For this review, take the finished solid that the model builds, in its own axes (mm). A direction names the side the tool comes from. Round coordinates to 2 decimals unless told otherwise and drop trailing zeros. Order: outer loops, then holes, each group sorted by start corner. A loop starts at its lowest first (then second) coordinate and runs counter-clockwise, first axis right, second up. Notation, with made-up numbers: (24, -15) - (67, -15) arc R8 ccw to (67, -7) - close; hole circle Ø1 at (67.5, 34). An arc over 180 degrees is marked (long way). Write each question's results on one line, items separated by ' | '. Start each with the question number.
(1) Take a section at D-D, the plane y = -23. Give the boundary of the cut face in (x, z), plus the area to 3 significant figures.
(2) For L1, parallel to Y at x = 42.25, z = 0.7; L2, parallel to X at y = -9.5, z = 2.9; L3, parallel to Y at x = 41, z = 3.05, list the stretches that pass through material, from the lowest coordinate up. Write a range as from..to.
(3) Take a section at A-A, the plane x = 42.25. Give the boundary of the cut face in (y, z).
(4) Draft analysis for pull direction Y (two halves, no side actions). For faces 4 (the flat face through (44, -4, 2)), 5 (the cylindrical face through (41.06, -34.91, 0.76)), 6 (the cylindrical face through (8.56, -34.91, 0.76)), 7 (the flat face through (23, -41, 3.5)), state which applies: pulls with the +Y half, pulls with the -Y half, needs draft (parallel to the pull), parting line crosses it, or undercut.
(5) For faces 1 (the flat face through (44, -42, 2)), 2 (the flat face through (17.5, -44, 3)), 3 (the flat face through (49, -24, 3.5)), list the 3-axis set-ups (+Z, -Z, +X, -X, +Y, -Y) from which the entire face can be reached by the end or side of a thin tool; tool diameter is ignored.
(6) Take a section at B-B, the plane y = -12. Give the boundary of the cut face in (x, z).
(7) Insertion check: pin 1 Ø1.2 at (y, z) = (-43, 2.5) entering from -X; pin 2 Ø1.6 at (y, z) = (-17.5, 2.5) entering from +X; pin 3 Ø3.5 at (x, y) = (26, -23) entering from +Z. Each pin has a flat end and moves straight along its axis. Give the tip position at first contact, or say it passes through.
(8) Take a section at C-C, the plane x = 26. Give the boundary of the cut face in (y, z).
```python
from build123d import *

# Parameters (mm, degrees)
F0_W      = 52
F0_H      = 46
F1_DEPTH  = 1.5
F2_W      = 48.5
F2_H      = 38
F2_W_2    = 44.5
F2_H_2    = 34
F3_DEPTH  = 2
F4_W      = 10
F4_H      = 4
F5_DEPTH  = 4
F6_R      = 1.5
F7_DEPTH  = 25
F8_DEPTH  = 2
F9_DEPTH  = 2
F10_DEPTH = 2
F11_DEPTH = 2


with BuildPart() as f1:
    # F0 (on Top) → F1 (new body)
    with BuildSketch(Plane.XY):
        with Locations((26, -23)):
            Rectangle(F0_W, F0_H)
    extrude(amount=F1_DEPTH)

    # F2 (on face) → F3 (join)
    with BuildSketch(Plane.XY.offset(1.5)):
        with Locations((26, -23)):
            Rectangle(F2_W, F2_H)
        with Locations((26, -23)):
            Rectangle(F2_W_2, F2_H_2, mode=Mode.SUBTRACT)
    extrude(amount=F3_DEPTH)

    # F4 (on face) → F5 (join)
    with BuildSketch(Plane.XY.offset(1.5)):
        with Locations((12.5, -44)):
            Rectangle(F4_W, F4_H)
        with Locations((33, -44)):
            Rectangle(F4_W, F4_H)
        with Locations((33, -2)):
            Rectangle(F4_W, F4_H)
        with Locations((12.5, -2)):
            Rectangle(F4_W, F4_H)
    extrude(amount=F5_DEPTH)

    # F6 (on face) → F7 (cut)
    with BuildSketch(Plane.XY.offset(1.5)):
        with Locations((9.75, -12)):
            Circle(F6_R)
        with Locations((42.25, -12)):
            Circle(F6_R)
        with Locations((26, -23)):
            Circle(F6_R)
        with Locations((9.75, -34)):
            Circle(F6_R)
        with Locations((42.25, -34)):
            Circle(F6_R)
    extrude(amount=-F7_DEPTH, mode=Mode.SUBTRACT)

    # F8 (add, through all): a face of the model
    f8_faces = [f1.faces().sort_by_distance(p)[0] for p in [
        (12.5, -4, 4.5),
    ]]
    extrude(f8_faces, amount=F8_DEPTH)

    # F9 (add, through all): a face of the model
    f9_faces = [f1.faces().sort_by_distance(p)[0] for p in [
        (33, -4, 4.5),
    ]]
    extrude(f9_faces, amount=F9_DEPTH)

    # F10 (add, through all): a face of the model
    f10_faces = [f1.faces().sort_by_distance(p)[0] for p in [
        (33, -42, 4.5),
    ]]
    extrude(f10_faces, amount=F10_DEPTH)

    # F11 (add, through all): a face of the model
    f11_faces = [f1.faces().sort_by_distance(p)[0] for p in [
        (12.5, -42, 4.5),
    ]]
    extrude(f11_faces, amount=F11_DEPTH)


solid = f1.part
```
Results below:
1) outline: (0, 0) - (24.5, 0) - (24.5, 1.5) - (3.75, 1.5) - (3.75, 3.5) - (1.75, 3.5) - (1.75, 1.5) - (0, 1.5) - close; (27.5, 0) - (52, 0) - (52, 1.5) - (50.25, 1.5) - (50.25, 3.5) - (48.25, 3.5) - (48.25, 1.5) - (27.5, 1.5) - close | area: 81.5 mm^2
2) L1: y = -46..-35.5, -32.5..-13.5, -10.5..0 | L2: x = 1.75..3.75, 48.25..50.25 | L3: y = -42..-40, -6..-4
3) outline: (-46, 0) - (-35.5, 0) - (-35.5, 1.5) - (-40, 1.5) - (-40, 3.5) - (-42, 3.5) - (-42, 1.5) - (-46, 1.5) - close; (-32.5, 0) - (-13.5, 0) - (-13.5, 1.5) - (-32.5, 1.5) - close; (-10.5, 0) - (0, 0) - (0, 1.5) - (-4, 1.5) - (-4, 3.5) - (-6, 3.5) - (-6, 1.5) - (-10.5, 1.5) - close
4) face 4: pulls with the +Y half | face 5: undercut | face 6: undercut | face 7: needs draft
5) face 1: +Z, +X, -Y | face 2: +Z, -Y | face 3: +Z, +X, +Y, -Y
6) outline: (0, 0) - (8.25, 0) - (8.25, 1.5) - (3.75, 1.5) - (3.75, 3.5) - (1.75, 3.5) - (1.75, 1.5) - (0, 1.5) - close; (11.25, 0) - (40.75, 0) - (40.75, 1.5) - (11.25, 1.5) - close; (43.75, 0) - (52, 0) - (52, 1.5) - (50.25, 1.5) - (50.25, 3.5) - (48.25, 3.5) - (48.25, 1.5) - (43.75, 1.5) - close
7) pin 1: stops at x = 7.5 | pin 2: stops at x = 50.25 | pin 3: stops at z = 1.5
8) outline: (-46, 0) - (-24.5, 0) - (-24.5, 1.5) - (-40, 1.5) - (-40, 3.5) - (-42, 3.5) - (-42, 1.5) - (-46, 1.5) - close; (-21.5, 0) - (0, 0) - (0, 1.5) - (-4, 1.5) - (-4, 3.5) - (-6, 3.5) - (-6, 1.5) - (-21.5, 1.5) - close
